Geometry check sheet. Reference: the model listing, model coordinates, mm. Round coordinates to 2 decimals unless told otherwise and drop trailing zeros. Write each loop counter-clockwise with the first axis right and the second up, starting at its lowest first coordinate (ties: lowest second). Pieces come first, ordered by that corner, then holes.
Item 1: Cross-section at B-B (z = -115). Enter the section's corners in (x, y) (1 decimal), then the cut area to 3 significant figures.
Item 2: Cross-section at C-C (x = 9.25). Enter the section's corners in (y, z) (3 decimals), then the cut area to 3 significant figures.
Item 3: Cross-section at D-D (z = 71). Enter the section's corners in (x, y) (3 decimals), then the cut area to 3 significant figures.
Item 4: Cross-section at A-A (y = -16). Enter the section's corners in (x, z) (3 decimals), then the cut area to 3 significant figures.
Item 5: Scan lines: probe 1 along Y at (x, z) = (0.8, 158.75); probe 2 along Y at (x, z) = (24.15, -115); probe 3 along X at (y, z) = (-8, -14) (3 decimals). Record each from-to range of solid material in increasing order.
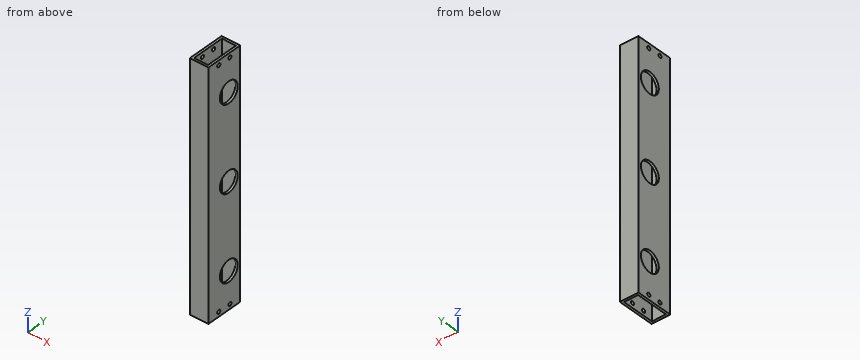
from build123d import *

# Parameters (mm, degrees)
SKETCH1_W                  = 330.2
SKETCH1_H                  = 50.8
SKETCH1_R                  = 14.2875
BOSS_EXTRUDE1_DEPTH        = 25.4
SHELL1_T                   = -3.175
F_9_0_196_DIAMETER_HOLE1_D = 4.9784


with BuildPart() as part:
    # Sketch1 → Boss-Extrude1 (new body)
    with BuildSketch(Plane(origin=(0, 0, 0), x_dir=(0, 0, -1), z_dir=(1, 0, 0))):
        Rectangle(SKETCH1_W, SKETCH1_H)
        with Locations((115, 7.112)):
            Circle(SKETCH1_R, mode=Mode.SUBTRACT)
        with Locations((-115, 7.112)):
            Circle(SKETCH1_R, mode=Mode.SUBTRACT)
        with Locations((0, 7.112)):
            Circle(SKETCH1_R, mode=Mode.SUBTRACT)
    extrude(amount=BOSS_EXTRUDE1_DEPTH)

    # Shell1
    shell1_openings = [part.faces().sort_by_distance(p)[0] for p in [
        (12.7, 0, -165.1),
        (12.7, 0, 165.1),
        (12.7, 7.112, 14.2875),
        (12.7, 7.112, 129.2875),
        (12.7, 7.112, -100.7125),
    ]]
    offset(amount=SHELL1_T, openings=shell1_openings, kind=Kind.INTERSECTION)

    # #9 (0.196) Diameter Hole1 (through all)
    with Locations(Plane(origin=(25.4, 0, 0), x_dir=(0, 0, -1), z_dir=(1, 0, 0))):
        with Locations((-158.75, 8.89), (-158.75, -8.89)):
            f_9_0_196_diameter_hole1 = Hole(F_9_0_196_DIAMETER_HOLE1_D / 2)

    # Mirror1: #9 (0.196) Diameter Hole1 across plane
    add(f_9_0_196_diameter_hole1.mirror(Plane.XY), mode=Mode.SUBTRACT)


solid = part.part
Resolved:
1. outline: (0, -25.4) - (25.4, -25.4) - (25.4, -7.2) - (22.2, -7.2) - (22.2, -22.2) - (3.2, -22.2) - (3.2, -7.2) - (0, -7.2) - close; (0, 21.4) - (3.2, 21.4) - (3.2, 22.2) - (22.2, 22.2) - (22.2, 21.4) - (25.4, 21.4) - (25.4, 25.4) - (0, 25.4) - close
1. area: 262 mm2
2. outline: (-25.4, -165.1) - (-22.225, -165.1) - (-22.225, 165.1) - (-25.4, 165.1) - close; (22.225, -165.1) - (25.4, -165.1) - (25.4, 165.1) - (22.225, 165.1) - close
2. area: 2,100 mm2
3. outline: (0, -25.4) - (25.4, -25.4) - (25.4, 25.4) - (0, 25.4) - close; hole (3.175, -22.225) - (22.225, -22.225) - (22.225, 22.225) - (3.175, 22.225) - close
3. area: 444 mm2
4. outline: (0, -165.1) - (3.175, -165.1) - (3.175, 165.1) - (0, 165.1) - close; (22.225, -165.1) - (25.4, -165.1) - (25.4, 165.1) - (22.225, 165.1) - close
4. area: 2,100 mm2
5. probe 1: y = -25.4 to -11.38, -6.4 to 6.4, 11.38 to 25.4
5. probe 2: y = -25.4 to -7.18, 21.4 to 25.4
5. probe 3: x = 0 to 3.175, 22.225 to 25.4
